Study the drawing (mm; zero at the part's minimum x, y, z) and answer. A direction names the side the tool comes from. Coordinates: 2 decimals unless noted, no trailing zeros. Order: outer loops, then holes, each group sorted by start corner. A loop starts at its lowest first (then second) coordinate and runs counter-clockwise, first axis right, second up. Notation, with made-up numbers: (15.25, 17) - (43.25, 17) arc R19 ccw to (43.25, 24) - close; hole circle Ø3 at (-34, 0.25). An arc over 180 degrees is marked (long way). Write item = value, one per line.
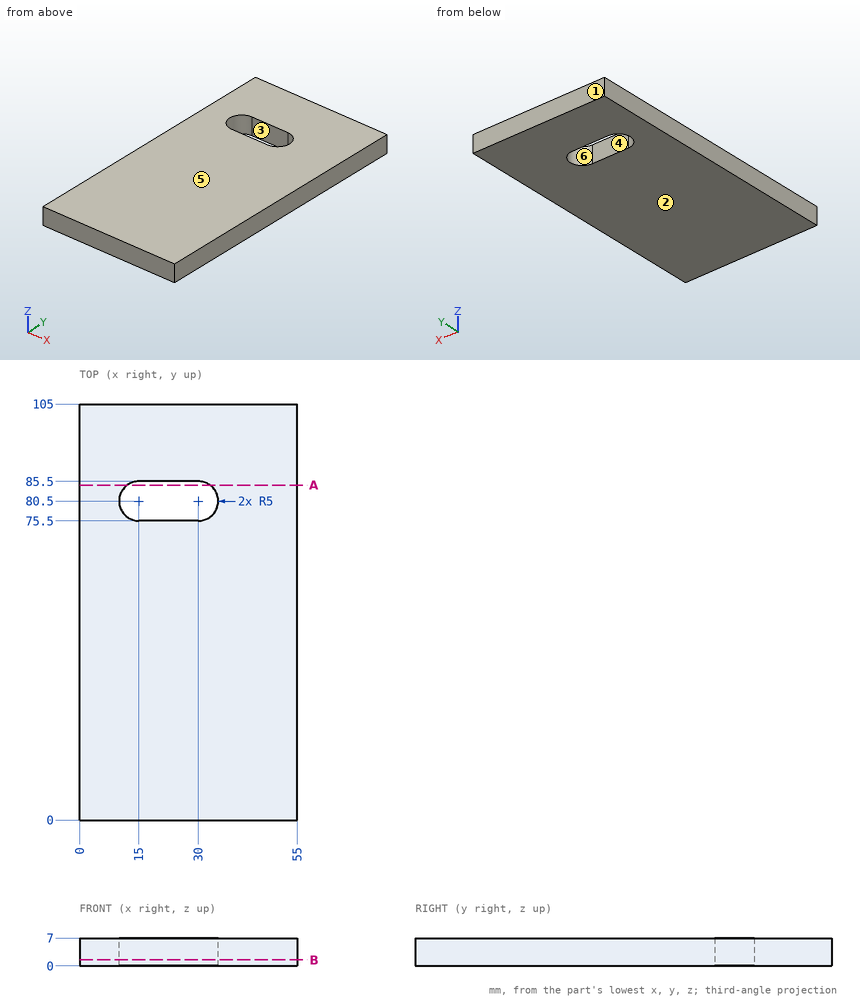
1) The part is cut by section B-B (z = 1.5). Determine the outline of the cut face in (x, y), and give its area (3 significant figures).
Returned:
outline = (0, 0) - (55, 0) - (55, 105) - (0, 105) - close; hole (15, 75.5) - (30, 75.5) arc R5 ccw to (30, 85.5) - (15, 85.5) arc R5 ccw to start
area = 5,550 mm^2
2) For the marked faces 5 and 6, determine the directions among +Z, -Z, +X, -X, +Y, -Y from which every point of the face is accessible in a straight line to the end or side of a thin tool.
Returned:
face_5 = +Z, +X, -X, +Y, -Y
face_6 = +Z, -Z
3) Determine the mould class of the marked faces 1, 2, 3 and 4 for opening direction Y: pulls with the +Y half, pulls with the -Y half, needs draft (parallel to the pull), parting line crosses it, or undercut.
Returned:
face_1 = pulls with the +Y half
face_2 = needs draft
face_3 = undercut
face_4 = undercut
4) The part is cut by section A-A (y = 84.5). Determine the outline of the cut face in (x, z).
Returned:
outline = (0, 0) - (12, 0) - (12, 7) - (0, 7) - close; (33, 0) - (55, 0) - (55, 7) - (33, 7) - close
5) Straight lines are drawn through the part: line 1 along Y through (x, z) = (16, 4.25); line 2 along X through (y, z) = (76, 2.25); line 3 along X through (y, z) = (78.5, 1.75). For each, find the intervals that lie inside material, in ascending order. Write a range as from..to.
Returned:
line_1 = 0..75.5, 85.5..105
line_2 = 0..12.82, 32.18..55
line_3 = 0..10.42, 34.58..55
